Here's how the part is built. I have some questions about the finished solid (model axes, mm). Face numbers are marked on the shaded views. Round coordinates to 2 decimals unless told otherwise and drop trailing zeros. Write each loop counter-clockwise with the first axis right and the second up, starting at its lowest first coordinate (ties: lowest second). Pieces come first, ordered by that corner, then holes. Notation, with made-up numbers: (18, 7) - (49, 7) arc R26 cw to (49, 43) - close; hole circle Ø10 at (-26, -8). An arc over 180 degrees is marked (long way). Write item = value, one per line. Start each with the question number.
Item 1: If we section it at C-C (x = 2): Please give me the cut outline in (y, z), and give its area (3 significant figures).
Item 2: If we section it at D-D (y = 1.6): Please give me the cut outline in (x, z).
Item 3: If I drill on line 1 along Y through (x, z) = (2, -0.1); line 2 along X through (y, z) = (0.1, 0); line 3 along X through (y, z) = (-0.5, -0.7), over which ranges is the centre line in solid material (lowest first)? Write a range as [from, to].
Item 4: If we section it at A-A (y = 0): Please give me the cut outline in (x, z).
Item 5: For P1, Ø1.5, axis at x = 9.5, z = 1, coming from the +Y side; P2, Ø1.8, axis at x = 2, y = 0, coming from the -Z side, each with a flat end and sliding along its axis, tell me the tip position at first contact or that it passes through.
Item 6: Thinking about a two-plate mould opening in Y: for the marked faces 1, 2 and 3, which applies, pulls with the +Y half, pulls with the -Y half, needs draft (parallel to the pull), parting line crosses it, or undercut?
Item 7: If we section it at B-B (z = 0): Please give me the cut outline in (x, y), and give its area (3 significant figures).
```python
from build123d import *

# Parameters (mm, degrees)
SKETCH1_R           = 2
BOSS_EXTRUDE1_DEPTH = 22
SKETCH2_R           = 1
CUT_EXTRUDE1_DEPTH  = 4
FILLET2_R           = 2


with BuildPart() as part:
    # Sketch1 → Boss-Extrude1 (new body)
    with BuildSketch(Plane(origin=(0, 0, 0), x_dir=(0, 0, -1), z_dir=(1, 0, 0))):
        Circle(SKETCH1_R)
    extrude(amount=BOSS_EXTRUDE1_DEPTH)

    # Sketch2 → Cut-Extrude1 (cut)
    with BuildSketch(Plane.XY.offset(2)):
        with Locations((2, 0)):
            Circle(SKETCH2_R)
    extrude(amount=-CUT_EXTRUDE1_DEPTH, mode=Mode.SUBTRACT)

    # Fillet2
    fillet2_edges = [part.edges().sort_by_distance(p)[0] for p in [
        (22, 0, 2),
    ]]
    fillet(fillet2_edges, radius=FILLET2_R)


solid = part.part
```
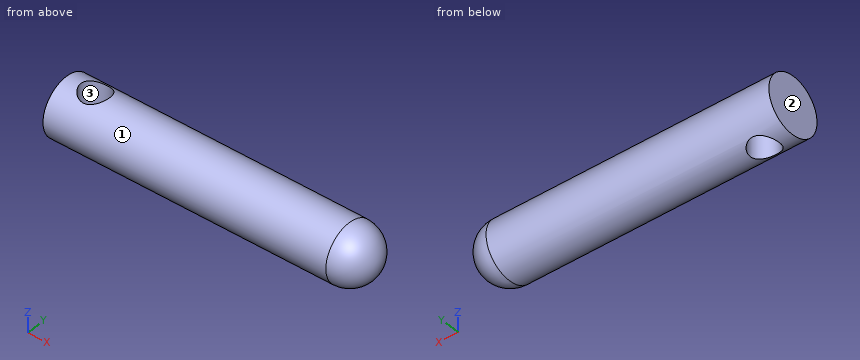
Reply:
q1.outline = (-1, -1.73) - (-1, 1.73) arc R2 ccw to start; (1, -1.73) arc R2 ccw to (1, 1.73) - close
q1.area = 4.91 mm2
q2.outline = (0, -1.2) - (20, -1.2) arc R1.2 ccw to (20, 1.2) - (0, 1.2) - close
q3.line_1 = [-2, -1], [1, 2]
q3.line_2 = [0, 1.01], [2.99, 22]
q3.line_3 = [0, 1.13], [2.87, 21.81]
q4.outline = (0, -2) - (1, -2) - (1, 2) - (0, 2) - close; (3, -2) - (20, -2) arc R2 ccw to (20, 2) - (3, 2) - close
q5.P1 = 1.98
q5.P2 = through
q6.face_1 = parting line crosses it
q6.face_2 = needs draft
q6.face_3 = undercut
q7.outline = (0, -2) - (20, -2) arc R2 ccw to (20, 2) - (0, 2) - close; hole circle Ø2 at (2, 0)
q7.area = 83.1 mm2
